Check sheet for the modelled part. Datum: model origin and axes. Units: mm. Round coordinates to 2 decimals unless told otherwise and drop trailing zeros. Write each loop counter-clockwise with the first axis right and the second up, starting at its lowest first coordinate (ties: lowest second). Pieces come first, ordered by that corner, then holes.
Item 1: Section check C-C, the plane x = -113. Record the cut outline in (y, z) (3 decimals).
Item 2: Material ranges on line 1 along Y through (x, z) = (-90, -0.5); line 2 along Y through (x, z) = (-86, 0); line 3 along Y through (x, z) = (-89, -2), recorded low to high.
Item 3: Section check A-A, the plane y = 0. Record the cut outline in (x, z) (1 decimal).
Item 4: Depth check by flat-ended pin: pin 1 (8 mm diameter, centred on x = -65.48, y = 21.48, fed in from +Z); pin 2 (8 mm diameter, centred on x = -125.73, y = 34.29, fed in from -Z) (3 decimals); pin 3 (1.5 mm diameter, centred on y = -64, z = -0.5, fed in from -X); pin 4 (6 mm diameter, centred on x = -98.65, y = 55.06, fed in from +Z). Enter the tip coordinate at first touch or a pass-through.
Item 5: Section check D-D, the plane y = -71.5. Record the cut outline in (x, z) (3 decimals).
Item 6: Section check B-B, the plane z = -2. State how many separate pieces and enclosed holes the cut face has, plus the area to 3 significant figures.
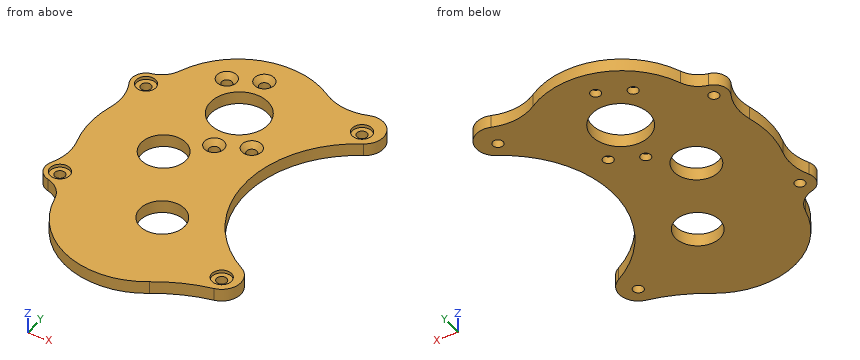
Autodesk Inventor part; units mm, degrees
ref_plane "YZ Plane" through (0, 0, 0) normal (1, 0, 0) x (0, 1, 0)
ref_plane "XZ Plane" through (0, 0, 0) normal (0, 1, 0) x (-1, 0, 0)
ref_plane "XY Plane" through (0, 0, 0) normal (0, 0, 1) x (1, 0, 0)
sketch "Sketch1" plane through (0, 0, 0) normal (0, 0, 1) x (1, 0, 0)
  circle A0 centre (0, 0) radius 53.975 construction
  circle A1 centre (-95.7467, 0) radius 11.1125
  circle A2 centre (-73.1257, -37.5239) radius 11.1125
  line L0 (-195.0218, 0) -> (95.4745, 0)
  line L1 (0, -186.751) -> (0, 135.7508)
  circle A3 centre (-82.0671, 38.2685) radius 14.2875
  arc A4 (-27.1037, 48.5034) -> (-27.1037, -48.5034) centre (0, 0) ccw
  arc A5 (-27.1037, 48.5034) -> (-34.976, 65.7804) centre (-31.75, 56.8183) ccw
  circle A6 centre (-95.7467, 0) radius 33.02 construction
  arc A7 (-57.3305, 68.3238) -> (-118.1642, 48.9464) centre (-79.7457, 33.5145) ccw
  arc A8 (-57.3305, 68.3238) -> (-34.976, 65.7804) centre (-43.5788, 89.6792) ccw
  arc A9 (-29.7745, -66.1362) -> (-27.1037, -48.5034) centre (-31.75, -56.8183) ccw
  arc A10 (-118.11, -50.8) -> (-55.2575, -76.6338) centre (-77.6901, -41.8358) ccw
  arc A11 (-29.7745, -66.1362) -> (-55.2575, -76.6338) centre (-13.9704, -140.6793) ccw
  circle A12 centre (-82.0671, 38.2685) radius 33.02 construction
  circle A13 centre (-73.1257, -37.5239) radius 39.37 construction
  circle A14 centre (-95.7467, 0) radius 10.16 construction
  circle A15 centre (0, 0) radius 16.51 construction
  circle A16 centre (-73.1257, -37.5239) radius 16.51 construction
  line L2 (0, 0) -> (-82.0671, 38.2685) construction
  circle A17 centre (-125.73, 34.29) radius 6.35 construction
  circle A18 centre (-125.73, -34.29) radius 6.35 construction
  line L3 (0, 0) -> (-34.976, 65.7804) construction
  line L4 (0, 0) -> (-57.3305, 68.3238) construction
  arc A19 (-127.2489, 41.2704) -> (-132.0785, 31.0144) centre (-125.73, 34.29) ccw
  arc A20 (-130.3268, 13.3001) -> (-130.3268, -13.3001) centre (-83.9357, 0) ccw
  arc A21 (-130.3268, 13.3001) -> (-132.0785, 31.0144) centre (-153.5223, 19.9501) ccw
  arc A22 (-132.0785, -31.0144) -> (-127.4503, -41.2235) centre (-125.73, -34.29) ccw
  arc A23 (-132.0785, -31.0144) -> (-130.3268, -13.3001) centre (-153.5223, -19.9501) ccw
  arc A24 (-118.11, -50.8) -> (-127.4503, -41.2235) centre (-130.5087, -53.5498) ccw
  arc A25 (-127.2489, 41.2704) -> (-118.1642, 48.9464) centre (-129.949, 53.6801) ccw
  line L5 (-118.1642, 48.9464) -> (0, 48.9464) construction
  line L6 (-118.11, -50.8) -> (0, -50.8) construction
  dimension "d0" = 107.95
  dimension "d9" = 22.225
  dimension "d38" = 28.575
  dimension "d63" = 1.5875
  dimension "d66" = 9.525
  dimension "d77" = 31.75
  dimension "d93" = 66.04
  dimension "d95" = 25.4
  dimension "d106" = 66.04
  dimension "d107" = 78.74
  dimension "d108" = 20.32
  dimension "d110" = 33.02
  dimension "d116" = 43.815
  dimension "d117" = 40.64
  dimension "d118" = 33.02
  dimension "d119" = 22.225
  dimension "d120" = 65
  dimension "d121" = 90.551
  dimension "d125" = 12.7
  dimension "d126" = 12.7
  dimension "d128" = 28
  dimension "d129" = 40
  dimension "d130" = 34.29
  dimension "d131" = 125.73
  dimension "d133" = 34.29
  dimension "d134" = 125.73
  dimension "d141" = 14.2875
  dimension "d144" = 14.2875
  dimension "d145" = 11.811
  dimension "d146" = 24.13
  dimension "d147" = 24.13
  dimension "d150" = 48.26
  dimension "d151" = 12.7
  dimension "d152" = 12.7
  dimension "d153" = 41.402
  dimension "d155" = 76.2
  dimension "d156" = 31.75
  dimension "d157" = 9.525
  dimension "d158" = 118.11
  dimension "d159" = 50.8
extrude "Base" add sketch "Sketch1" along normal mid plane 6.35 contours L0 A4 A9 A11 A10 A24 A22 A23 A20 A1 | A1 L0 A20 A21 A19 A25 A7 A8 A5 A4
sketch "Sketch4" plane through (0, 0, 3.175) normal (0, 0, 1) x (1, 0, 0)
  circle A0 centre (-82.0671, 38.2685) radius 14.2875
  line L0 (-98.6536, 55.0567) -> (-84.2659, 61.7657) construction
  line L1 (-79.8682, 14.7713) -> (-65.4806, 21.4803) construction
  line L2 (-155.0035, 0) -> (-0.0953, 0)
  line L3 (0, -114.8687) -> (0, 106.5474)
  line L4 (-72.6744, 18.1258) -> (-91.4598, 58.4112) construction
  point P0 (-82.0671, 38.2685)
  dimension "d122" = 15.875
  dimension "d123" = 44.45
  dimension "d124" = 25
hole "Encoder Mount Holes" at (-98.6536, 55.0567, 3.175) at (-84.2659, 61.7657, 3.175) at (-79.8682, 14.7713, 3.175) at (-65.4806, 21.4803, 3.175) direction (0, 0, -1) diameter 5.1054 end through all countersink diameter 9.779 countersink angle 82
sketch "Sketch5" plane through (0, 0, 3.175) normal (0, 0, 1) x (1, 0, 0)
  arc A0 (-27.1037, 48.5034) -> (-27.1037, -48.5034) centre (0, 0) ccw
  line L0 (0, 0) -> (-31.75, 54.9926) construction
  line L1 (-159.4485, 0) -> (26.5747, 0) construction
  line L2 (0, -114.8687) -> (0, 106.5474) construction
  line L3 (-30.9294, -58.1697) -> (0, 0) construction
  dimension "d64" = 30
  dimension "d65" = 63.5
  dimension "d100" = 65.8812
  dimension "d102" = 62
hole "Standoff holes to motor plate" at (-31.75, 54.9926, 3.175) at (-30.9294, -58.1697, 3.175) direction (0, 0, -1) diameter 5.1054 end through all counterbore diameter 9.779 counterbore depth 1.5875
sketch "Sketch7" plane through (0, 0, 3.175) normal (0, 0, 1) x (1, 0, 0)
  arc A0 (-127.2489, 41.2704) -> (-132.0785, 31.0144) centre (-125.73, 34.29) ccw
  arc A1 (-132.0785, -31.0144) -> (-127.4503, -41.2235) centre (-125.73, -34.29) ccw
hole "Standoff holes to front plate" at (-125.73, 34.29, 3.175) at (-125.73, -34.29, 3.175) direction (0, 0, -1) diameter 5.1054 end through all counterbore diameter 9.779 counterbore depth 1.5875
properties part number "connected plate"
Values found:
1. outline: (-63.454, -3.175) - (58.178, -3.175) - (58.178, 3.175) - (-63.454, 3.175) - close
2. line 1: y = -81.37 to -9.51, 9.51 to 26.39, 50.15 to 73.63
2. line 2: y = -82.4 to -5.34, 5.34 to 24.53, 52 to 59.89, 63.64 to 74.44
2. line 3: y = -81.66 to -8.83, 8.83 to 25.78, 50.76 to 73.87
3. outline: (-132.2, -3.2) - (-106.9, -3.2) - (-106.9, 3.2) - (-132.2, 3.2) - close; (-84.6, -3.2) - (-55.6, -3.2) - (-55.6, 3.2) - (-84.6, 3.2) - close
4. pin 1: stops at z = 2.15
4. pin 2: stops at z = -3.175
4. pin 3: stops at x = -113.12
4. pin 4: stops at z = 1.01
5. outline: (-106.572, -3.175) - (-45.918, -3.175) - (-45.918, 3.175) - (-106.572, 3.175) - close
6. separate pieces: 1
6. enclosed holes: 11
6. area: 10,700 mm2
